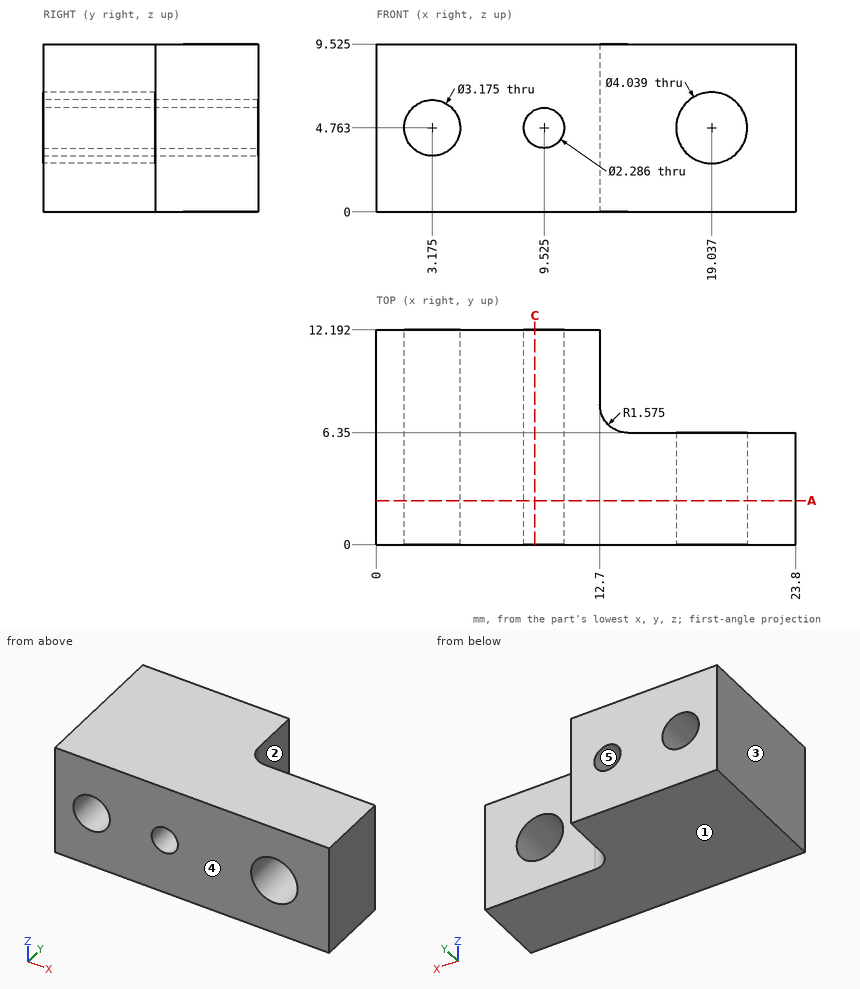
Can you work these out from the drawing? Everything is in mm from the part's minimum corner. A direction names the side the tool comes from. Give positions to 0.01 mm unless a question says otherwise; leave off trailing zeros. Order: outer loops, then holes, each group sorted by start corner. A loop starts at its lowest first (then second) coordinate and runs counter-clockwise, first axis right, second up.
1. Suppose I cut it at A-A (y = 2.5). Give the number of separate pieces and of enclosed holes in the cut face, plus the area to 3 significant figures.
2. We'd pull the mould along X, two halves only. Please class the marked faces 3, 4 and 5: pulls with the +X half, pulls with the -X half, needs draft (parallel to the pull), parting line crosses it, or undercut.
3. Suppose I cut it at C-C (x = 9). List the corners of the cut face in (y, z) for me (1 decimal).
4. Will these pins go through, and if not, where does the flat tip stop? P1, Ø2, axis at x = 4.5, z = 4, coming from the +Y side; P2, Ø1, axis at y = 7.5, z = 6, coming from the +X side; P3, Ø3.5, axis at y = 9.5, z = 6, coming from the +X side.
5. I need wall thicknesses on L1, parallel to X at y = 11.25, z = 5.25 (1 decimal); L2, parallel to X at y = 6, z = 6 (1 decimal); L3, parallel to X at y = 4, z = 4.25 (1 decimal). Which ranges of each line are inside material? Lowest first, please.
6. For the marked faces 1 and 2, which set-ups out of +Z, -Z, +X, -X, +Y, -Y let a thin tool reach every point of the face, with its end or its side?
Solved:
1. separate pieces: 1
1. enclosed holes: 3
1. area: 202 mm2
2. face 3: pulls with the -X half
2. face 4: needs draft
2. face 5: undercut
3. outline: (0, 0) - (12.2, 0) - (12.2, 3.7) - (0, 3.7) - close; (0, 5.8) - (12.2, 5.8) - (12.2, 9.5) - (0, 9.5) - close
4. P1: stops at y = 12.19
4. P2: stops at x = 13
4. P3: stops at x = 12.71
5. L1: x = 0 to 1.7, 4.7 to 8.5, 10.6 to 12.7
5. L2: x = 0 to 2.2, 4.2 to 17.4, 20.6 to 23.8
5. L3: x = 0 to 1.7, 4.7 to 8.5, 10.5 to 17.1, 21 to 23.8
6. face 1: -Z, +X, -X, +Y, -Y
6. face 2: +Z, -Z, +X, +Y
